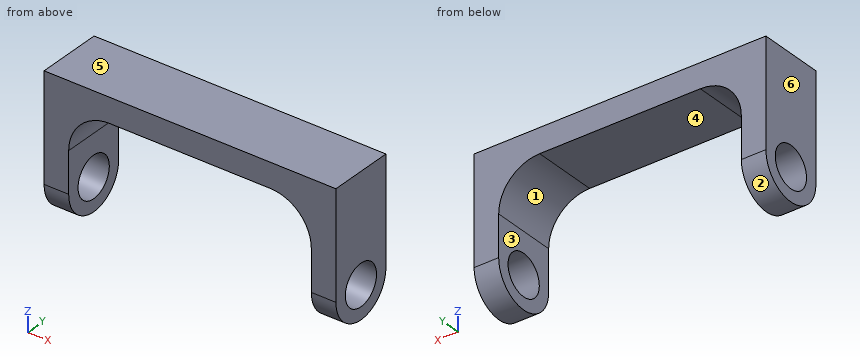
from build123d import *

# Parameters (mm, degrees)
BOSS_EXTRUDE1_START = -0.5
SKETCH2_W           = 3
SKETCH2_H           = 8
SKETCH2_R           = 2.5
BOSS_EXTRUDE1_DEPTH = 3
BOSS_EXTRUDE2_START = 2.5
SKETCH2_3_W         = 3
SKETCH2_3_H         = 8
BOSS_EXTRUDE2_DEPTH = 29.6
BOSS_EXTRUDE3_START = 32.1
SKETCH2_4_W         = 3
SKETCH2_4_H         = 8
SKETCH2_4_R         = 2.5
BOSS_EXTRUDE3_DEPTH = 3
FILLET1_R           = 5


with BuildPart() as part:
    # Sketch2 → Boss-Extrude1 (new body)
    # profile 1 of 2: a face of its own
    with BuildSketch(Plane(origin=(0, 0, 0), x_dir=(0, 0, -1), z_dir=(1, 0, 0)).offset(BOSS_EXTRUDE1_START)):
        with Locations((-11.5, 0)):
            Rectangle(SKETCH2_W, SKETCH2_H)
    # profile 2 of 2: a face of its own
    with BuildSketch(Plane(origin=(0, 0, 0), x_dir=(0, 0, -1), z_dir=(1, 0, 0)).offset(BOSS_EXTRUDE1_START)):
        with BuildLine():
            Line((0, -4), (-10, -4))
            Line((-10, -4), (-10, 4))
            Line((-10, 4), (0, 4))
            ThreePointArc((0, 4), (4, 0), (0, -4))
        make_face()
        Circle(SKETCH2_R, mode=Mode.SUBTRACT)
    extrude(amount=BOSS_EXTRUDE1_DEPTH)

    # Sketch2<3> → Boss-Extrude2 (add)
    with BuildSketch(Plane(origin=(0, 0, 0), x_dir=(0, 0, -1), z_dir=(1, 0, 0)).offset(BOSS_EXTRUDE2_START)):
        with Locations((-11.5, 0)):
            Rectangle(SKETCH2_3_W, SKETCH2_3_H)
    extrude(amount=BOSS_EXTRUDE2_DEPTH)

    # Sketch2<4> → Boss-Extrude3 (add)
    # profile 1 of 2: a face of its own
    with BuildSketch(Plane(origin=(0, 0, 0), x_dir=(0, 0, -1), z_dir=(1, 0, 0)).offset(BOSS_EXTRUDE3_START)):
        with Locations((-11.5, 0)):
            Rectangle(SKETCH2_4_W, SKETCH2_4_H)
    # profile 2 of 2: a face of its own
    with BuildSketch(Plane(origin=(0, 0, 0), x_dir=(0, 0, -1), z_dir=(1, 0, 0)).offset(BOSS_EXTRUDE3_START)):
        with BuildLine():
            Line((0, -4), (-10, -4))
            Line((-10, -4), (-10, 4))
            Line((-10, 4), (0, 4))
            ThreePointArc((0, 4), (4, 0), (0, -4))
        make_face()
        Circle(SKETCH2_4_R, mode=Mode.SUBTRACT)
    extrude(amount=BOSS_EXTRUDE3_DEPTH)

    # Fillet1
    fillet1_edges = [part.edges().sort_by_distance(p)[0] for p in [
        (32.1, 0, 10),
        (2.5, 0, 10),
    ]]
    fillet(fillet1_edges, radius=FILLET1_R)


solid = part.part
Check sheet for the modelled part. Datum: model origin and axes. Units: mm. Face numbers are marked on the shaded views. A direction names the side the tool comes from. Give positions to 0.01 mm unless a question says otherwise; leave off trailing zeros. Write each loop counter-clockwise with the first axis right and the second up, starting at its lowest first coordinate (ties: lowest second). Pieces come first, ordered by that corner, then holes. Notation, with made-up numbers: M 0,8.5 L 26,8.5 A14 ccw 26,30.5 Z; hole C 83,-35.75 d7. An arc over 180 degrees is marked long. Use one line per item in the form item = value.
(1) Section check D-D on y = -3.25. Record the boundary of the cut face in (x, z).
Answer block:
outline = M -0.5,-2.33 L 2.5,-2.33 L 2.5,5 A5 cw 7.5,10 L 27.1,10 A5 cw 32.1,5 L 32.1,-2.33 L 35.1,-2.33 L 35.1,13 L -0.5,13 Z
(2) Section check C-C on z = 9. Record the boundary of the cut face in (x, y).
Answer block:
outline = M -0.5,-4 L 4.5,-4 L 4.5,4 L -0.5,4 Z; M 30.1,-4 L 35.1,-4 L 35.1,4 L 30.1,4 Z
(3) Tool access check on the marked faces 1 and 2. Record the directions out of +Z, -Z, +X, -X, +Y, -Y that give a thin tool (end or side, any length) a straight path to the whole face; none if there is none.
Answer block:
face_1 = -Z, +Y, -Y
face_2 = -Z, +X, -X
(4) Draft check along X on the marked faces 3, 4, 5 and 6. Enter one of: pulls with the +X half, pulls with the -X half, needs draft (parallel to the pull), parting line crosses it, or undercut.
Answer block:
face_3 = undercut
face_4 = undercut
face_5 = needs draft
face_6 = pulls with the -X half
(5) Section check B-B on y = 0. Record the boundary of the cut face in (x, z).
Answer block:
outline = M -0.5,-4 L 2.5,-4 L 2.5,-2.5 L -0.5,-2.5 Z; M -0.5,2.5 L 2.5,2.5 L 2.5,5 A5 cw 7.5,10 L 27.1,10 A5 cw 32.1,5 L 32.1,2.5 L 35.1,2.5 L 35.1,13 L -0.5,13 Z; M 32.1,-4 L 35.1,-4 L 35.1,-2.5 L 32.1,-2.5 Z
(6) Depth check by flat-ended pin: P1, Ø10, axis at x = 6, z = -0.5, coming from the +Y side. Enter the tip coordinate at first touch or a pass-through.
Answer block:
P1 = 4
(7) Section check A-A on z = 1.5. Record the boundary of the cut face in (x, y).
Answer block:
outline = M -0.5,-4 L 2.5,-4 L 2.5,-2 L -0.5,-2 Z; M -0.5,2 L 2.5,2 L 2.5,4 L -0.5,4 Z; M 32.1,-4 L 35.1,-4 L 35.1,-2 L 32.1,-2 Z; M 32.1,2 L 35.1,2 L 35.1,4 L 32.1,4 Z
(8) Material ranges on line 1 along Y through (x, z) = (1.2, 0); line 2 along X through (y, z) = (-3, 2.25); line 3 along Z through (x, y) = (19, -3.5), recorded low to high.
Answer block:
line_1 = -4 to -2.5, 2.5 to 4
line_2 = -0.5 to 2.5, 32.1 to 35.1
line_3 = 10 to 13
